Can you work these out from the model? Positions are in its coordinate system, mm. A direction names the side the tool comes from. Coordinates: 2 decimals unless noted, no trailing zeros. Order: outer loops, then holes, each group sorted by start corner. A loop starts at its lowest first (then second) coordinate and runs counter-clockwise, first axis right, second up. Notation, with made-up numbers: (58.25, 61) -> (85.25, 61) arc R32 ccw to (85.25, 97) -> close; hole circle Ø7 at (60, -17.75). An arc over 180 degrees is marked (long way). Write item = value, one per line.
Autodesk Inventor part; units mm, degrees
ref_plane "YZ Plane" through (0, 0, 0) normal (1, 0, 0) x (0, 1, 0)
ref_plane "XZ Plane" through (0, 0, 0) normal (0, 1, 0) x (-1, 0, 0)
ref_plane "XY Plane" through (0, 0, 0) normal (0, 0, 1) x (1, 0, 0)
sketch "スケッチ1" plane through (0, 0, 0) normal (0, 0, 1) x (1, 0, 0)
  line L0 (0, 0) -> (10, 0)
  line L1 (10, 0) -> (10, 10)
  line L2 (10, 10) -> (0, 10)
  line L3 (0, 10) -> (0, 0)
  dimension "d0" = 10
  dimension "d1" = 10
extrude "押し出し1" add sketch "スケッチ1" along normal blind 300
sketch "スケッチ2" plane through (0, 0, 300) normal (0, 0, 1) x (1, 0, 0)
  line L0 (1, 9) -> (9, 9)
  line L1 (9, 9) -> (9, 1)
  line L2 (9, 1) -> (1, 1)
  line L3 (1, 1) -> (1, 9)
  line L4 (10, 10) -> (0, 10)
  line L5 (10, 0) -> (10, 10)
  line L6 (0, 0) -> (10, 0)
  line L7 (0, 10) -> (0, 0)
  dimension "d4" = 1
  dimension "d5" = 1
  dimension "d6" = 1
  dimension "d7" = 1
extrude "押し出し2" cut sketch "スケッチ2" against normal through all contours L0 L1 L2 L3
sketch "スケッチ3" plane through (10, 0, 0) normal (1, 0, 0) x (0, 0, -1)
  line L0 (0, 0) -> (0, 10)
  point P0 (-15, 5)
  dimension "d10" = 15
hole "穴1" at (10, 5, 15) direction (-1, 0, 0) diameter 4 end through all
sketch "スケッチ4" plane through (10, 0, 0) normal (1, 0, 0) x (0, 0, -1)
  line L0 (0, 0) -> (0, 10)
  line L1 (0, 0) -> (-300, 0)
  point P0 (-5, 5)
  point P1 (-25, 5)
  dimension "d18" = 5
  dimension "d19" = 5
  dimension "d20" = 25
hole "穴2" at (10, 5, 5) at (10, 5, 25) direction (-1, 0, 0) diameter 3.5 end through all
properties part number "3SR06_振子"
Item 1: I want a section at B-B, the plane z = 72.5. Please give me the cut outline in (x, y).
A:
outline = (0, 0) -> (10, 0) -> (10, 10) -> (0, 10) -> close; hole (1, 1) -> (9, 1) -> (9, 9) -> (1, 9) -> close
Item 2: I want a section at A-A, the plane y = 5. Give the number of separate pieces and of enclosed holes in the cut face, plus the area to 3 significant figures.
A:
separate_pieces = 8
enclosed_holes = 0
area = 578 mm2
Item 3: For faces 1 (the flat face through (0, 5, 148)), 2 (the flat face through (5, 1, 152)), which set-ups out of +Z, -Z, +X, -X, +Y, -Y let a thin tool reach every point of the face, with its end or its side?
A:
face_1 = +Z, -Z, -X, +Y, -Y
face_2 = +Z, -Z
Item 4: If I drill on probe 1 along Y at (x, z) = (9.55, 5); probe 2 along Z at (x, y) = (9.2, 5); probe 3 along Y at (x, z) = (0.3, 15), over which ranges is the centre line in solid material (lowest first)?
A:
probe_1 = 0 to 3.25, 6.75 to 10
probe_2 = 0 to 3.25, 6.75 to 13, 17 to 23.25, 26.75 to 300
probe_3 = 0 to 3, 7 to 10
Item 5: I'm going to push a flat-ended pin straight in: P1, Ø3, axis at y = 5, z = 5, coming from the -X side. Where does the tip first touch, or does it pass through?
A:
P1 = through
Item 6: If we mould it in two halves opening along Y, with no side actions, what happens to faces 3 (the flat face through (1, 5, 152)), 4 (the flat face through (5, 10, 148)), 5 (the flat face through (5, 0, 148))? For each: pulls with the +Y half, pulls with the -Y half, needs draft (parallel to the pull), parting line crosses it, or undercut.
A:
face_3 = undercut
face_4 = pulls with the +Y half
face_5 = pulls with the -Y half
